Here's the drawing with two shaded views (mm, measured from the low corner). I have some questions. A direction names the side the tool comes from. Give positions to 0.01 mm unless a question says otherwise; leave off trailing zeros. Loops run counter-clockwise (first coordinate to the right, second up) from the corner with the lowest first, then second, coordinate; pieces in that order, holes last. Notation, with made-up numbers: M -27,-29.75 L 27,-29.75 A22 cw 27,-10.75 Z; hole C 8.5,24.25 d5. An arc over 180 degrees is marked long. Write item = value, one per line. Start each with the question number.
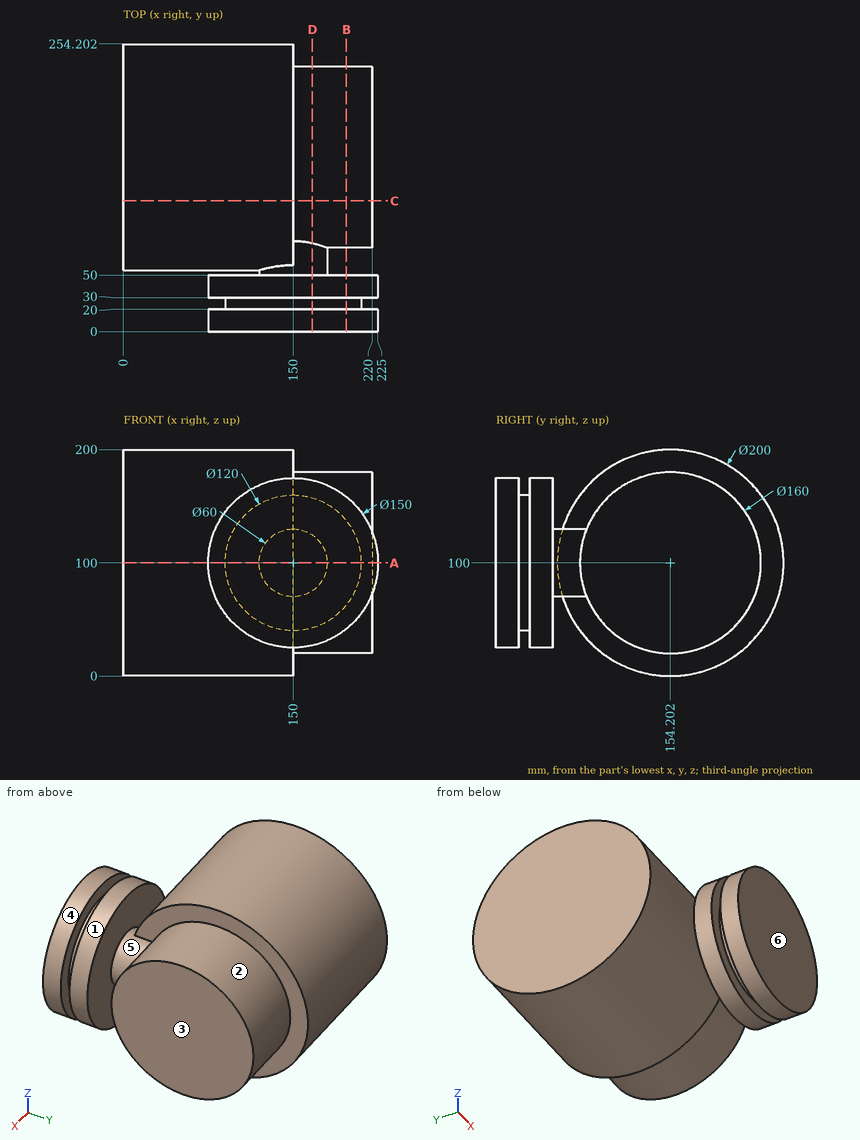
Q1. If we section it at B-B, the plane x = 197: List the corners of the cut face in (y, z) for me, then the cut area to 3 significant figures.
Q2. Will these pins go through, and if not, where does the flat tip stop? pin 1 (12 mm diameter, centred on y = 199.5, z = 21, fed in from +X); pin 2 (1.5 mm diameter, centred on x = 167.5, y = 128, fed in from -Z); pin 3 (10 mm diameter, centred on y = 49, z = 92.5, fed in from +X).
Q3. If we section it at A-A, the plane z = 100: List the corners of the cut face in (x, y) for me.
Q4. If we section it at D-D, the plane x = 167: List the corners of the cut face in (y, z) for me.
Q5. If I drill on line 1 along Y through (x, z) = (115, 37.5) (1 decimal); line 2 along X through (y, z) = (109, 137.5); line 3 along Y through (x, z) = (184, 120.5), over which ranges is the centre line in solid material (lowest first)?
Q6. If we section it at C-C, the plane y = 115.5: List the corners of the cut face in (x, z) for me.
Q7. On a 3-axis mill with a long thin cutter (end or side, diameter ignored), from which of +Z, -Z, +X, -X, +Y, -Y can I reach the whole of each face in a straight line? I mean the marked faces 1, 2 and 3. Say none if no direction works.
Q8. We'd pull the mould along Y, two halves only. Please class the marked faces 4, 5 and 6: pulls with the +Y half, pulls with the -Y half, needs draft (parallel to the pull), parting line crosses it, or undercut.
Resolved:
q1.outline = M 0,41.55 L 20,41.55 L 20,62.7 L 30,62.7 L 30,41.55 L 50,41.55 L 50,158.45 L 30,158.45 L 30,137.3 L 20,137.3 L 20,158.45 L 0,158.45 Z; C 154.2,100 d160
q1.area = 25,500 mm²
q2.pin_1 = 150
q2.pin_2 = 24.16
q2.pin_3 = 224.96
q3.outline = M 0,54.2 L 120,54.2 L 120,50 L 75,50 L 75,30 L 90,30 L 90,20 L 75,20 L 75,0 L 225,0 L 225,20 L 210,20 L 210,30 L 225,30 L 225,50 L 180,50 L 180,74.2 L 220,74.2 L 220,234.2 L 150,234.2 L 150,254.2 L 0,254.2 Z
q4.outline = M 0,26.95 L 20,26.95 L 20,42.46 L 30,42.46 L 30,26.95 L 50,26.95 L 50,75.28 L 78.12,75.28 A80 ccw long 78.12,124.72 L 50,124.72 L 50,173.05 L 30,173.05 L 30,157.54 L 20,157.54 L 20,173.05 L 0,173.05 Z
q5.line_1 = 0 to 20, 30 to 50, 76.1 to 232.3
q5.line_2 = 0 to 220
q5.line_3 = 0 to 50, 76.87 to 231.53
q6.outline = M 0,7.79 L 150,7.79 L 150,29.98 L 220,29.98 L 220,170.02 L 150,170.02 L 150,192.21 L 0,192.21 Z
q7.face_1 = -Y
q7.face_2 = +X
q7.face_3 = +Z, -Z, +X, +Y
q8.face_4 = needs draft
q8.face_5 = undercut
q8.face_6 = pulls with the -Y half
